Geometry check sheet. Reference: the model listing, model coordinates, mm. Face numbers are marked on the shaded views. A direction names the side the tool comes from. Give positions to 0.01 mm unless a question says otherwise; leave off trailing zeros. Loops run counter-clockwise (first coordinate to the right, second up) from the corner with the lowest first, then second, coordinate; pieces in that order, holes last. Notation, with made-up numbers: (-1.75, 9.25) -> (51.25, 9.25) arc R10 ccw to (51.25, 14.25) -> close; hole circle Ø9 at (38.5, 62). An arc over 180 degrees is marked (long way). One line per item, written item: value. Start each with the question number.
(1) Sectioned sample at B-B, the plane y = -30. Record the cut outline in (x, z).
(2) Tool access check on the marked faces 1 and 2. Record the directions out of +Z, -Z, +X, -X, +Y, -Y that give a thin tool (end or side, any length) a straight path to the whole face; none if there is none.
(3) Sectioned sample at D-D, the plane x = 6. Record the cut outline in (y, z), then the cut area to 3 significant figures.
(4) Sectioned sample at A-A, the plane z = 15. Record the cut outline in (x, y), then the cut area to 3 significant figures.
(5) Gauge pin test, flat ends, axial feed: pin 1 Ø5 at (y, z) = (-22.4, -23) entering from +X; pin 2 Ø5 at (x, z) = (-2.31, 15) entering from -Y. Record the tip position at first contact, or that the pin passes through.
(6) Scan lines: line 1 along Y through (x, z) = (-28, 0); line 2 along Y through (x, z) = (6, -8); line 3 along X through (y, z) = (-28, 13). Record each from-to range of solid material in increasing order. Write a range as from..to.
(7) Sectioned sample at C-C, the plane z = 0. State how many separate pieces and enclosed holes the cut face has, then the cut area to 3 significant figures.
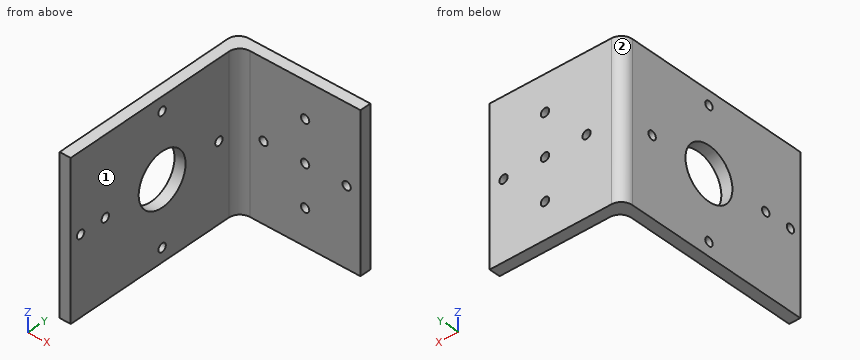
from build123d import *

# Parameters (mm, degrees)
BOSS_EXTRUDE1_DEPTH      = 28
BOSS_EXTRUDE1_DEPTH_BACK = 28
SKETCH3_R                = 9.5
SKETCH3_R_2              = 1.5
CUT_EXTRUDE1_DEPTH       = 4
FILLET2_R                = 4
SKETCH4_R                = 1.5
CUT_EXTRUDE2_DEPTH       = 4


with BuildPart() as part:
    # Sketch2 → Boss-Extrude1 (new body, two sides)
    with BuildSketch(Plane.XY) as boss_extrude1_sk:
        Polygon((-30.306244844, -59.398325359), (-26.306244844, -59.398325359), (-26.306244844, 8.601674641), (17.693755156, 8.601674641), (17.693755156, 12.601674641), (-30.306244844, 12.601674641), align=None)
    extrude(amount=BOSS_EXTRUDE1_DEPTH)
    extrude(boss_extrude1_sk.sketch, amount=-BOSS_EXTRUDE1_DEPTH_BACK)

    # Sketch3 → Cut-Extrude1 (cut)
    with BuildSketch(Plane(origin=(-26.306244844, 0, 0), x_dir=(0, 0, -1), z_dir=(1, 0, 0))):
        with Locations((0, -22.398325359)):
            Circle(SKETCH3_R)
        with Locations((0, 0.601674641)):
            Circle(SKETCH3_R_2)
        with Locations((23, -22.398325359)):
            Circle(SKETCH3_R_2)
        with Locations((0, -45.398325359)):
            Circle(SKETCH3_R_2)
        with Locations((-23, -22.398325359)):
            Circle(SKETCH3_R_2)
        with Locations((0, -55.398325359)):
            Circle(SKETCH3_R_2)
    extrude(amount=-CUT_EXTRUDE1_DEPTH, mode=Mode.SUBTRACT)

    # Fillet2
    fillet2_edges = [part.edges().sort_by_distance(p)[0] for p in [
        (-30.306244844, 12.601674641, 0),
        (-26.306244844, 8.601674641, 0),
    ]]
    fillet(fillet2_edges, radius=FILLET2_R)

    # Sketch4 → Cut-Extrude2 (cut)
    with BuildSketch(Plane.XZ.offset(-8.601674641)):
        with Locations((-2.306244844, 0)):
            Circle(SKETCH4_R)
        with Locations((-17.306244844, 0)):
            Circle(SKETCH4_R)
        with Locations((-2.306244844, 15)):
            Circle(SKETCH4_R)
        with Locations((12.693755156, 0)):
            Circle(SKETCH4_R)
        with Locations((-2.306244844, -15)):
            Circle(SKETCH4_R)
    extrude(amount=-CUT_EXTRUDE2_DEPTH, mode=Mode.SUBTRACT)


solid = part.part
Calculated:
1. outline: (-30.31, -28) -> (-26.31, -28) -> (-26.31, -5.7) -> (-30.31, -5.7) -> close; (-30.31, 5.7) -> (-26.31, 5.7) -> (-26.31, 28) -> (-30.31, 28) -> close
2. face 1: +Z, -Z, +X, -Y
2. face 2: +Z, -Z, -X, +Y
3. outline: (8.6, -28) -> (12.6, -28) -> (12.6, 28) -> (8.6, 28) -> close
3. area: 224 mm2
4. outline: (-30.31, -59.4) -> (-26.31, -59.4) -> (-26.31, 4.6) arc R4 cw to (-22.31, 8.6) -> (-3.81, 8.6) -> (-3.81, 12.6) -> (-26.31, 12.6) arc R4 ccw to (-30.31, 8.6) -> close; (-0.81, 8.6) -> (17.69, 8.6) -> (17.69, 12.6) -> (-0.81, 12.6) -> close
4. area: 452 mm2
5. pin 1: stops at x = -26.31
5. pin 2: stops at y = 8.6
6. line 1: y = -59.4..-56.9, -53.9..-46.9, -43.9..-31.9, -12.9..-0.9, 2.1..12.23
6. line 2: y = 8.6..12.6
6. line 3: x = -30.31..-26.31
7. separate pieces: 8
7. enclosed holes: 0
7. area: 316 mm2
